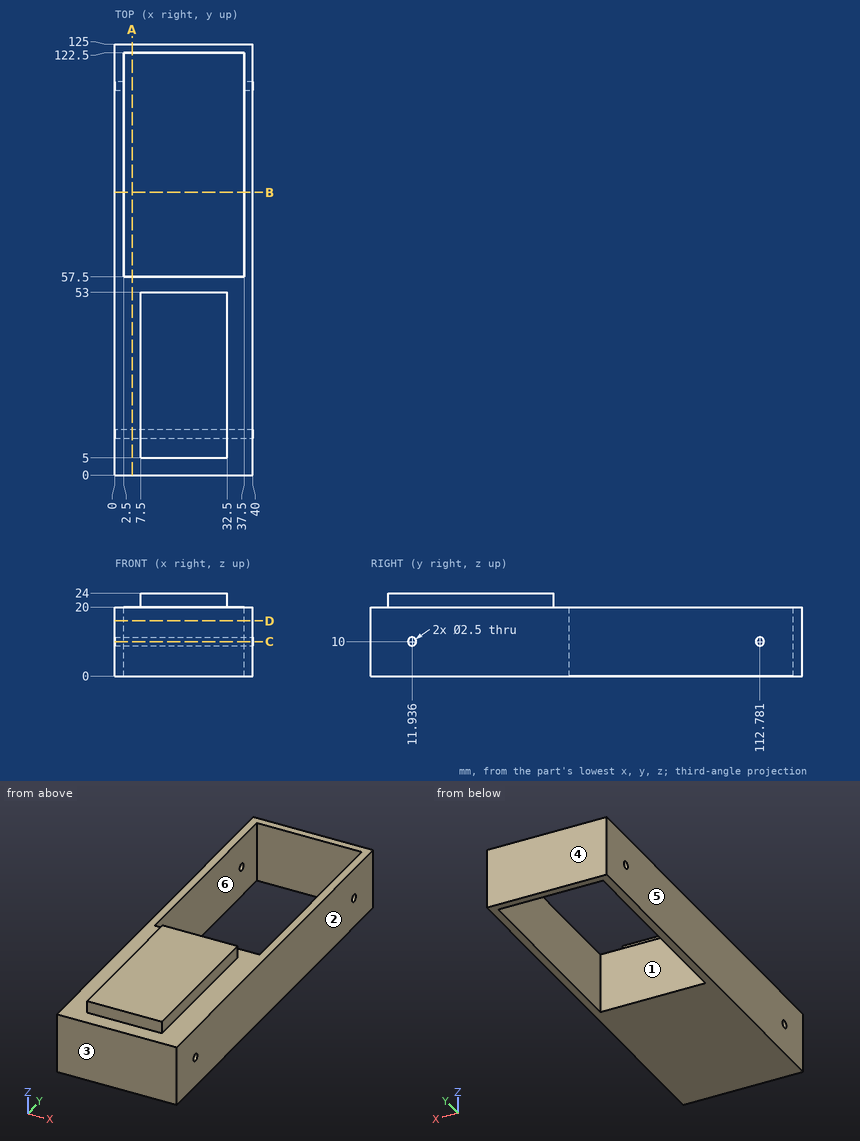
Could you check a few things on this drawing? It's one solid part, dimensions in mm from its lowest x, y, z. A direction names the side the tool comes from. Give positions to 0.01 mm unless a question says otherwise; leave off trailing zeros. Order: outer loops, then holes, each group sorted by start corner. A loop starts at its lowest first (then second) coordinate and runs counter-clockwise, first axis right, second up.
1. Thinking about a two-plate mould opening in Y: for the marked faces 3, 4, 5 and 6, which applies, +Y half, -Y half, draft (parallel to the pull), parting line (faces both ways), or undercut?
Answers below:
face 3: -Y half
face 4: +Y half
face 5: draft
face 6: undercut
2. Suppose I cut it at B-B (y = 82). Write out the boundary of the cut face in (x, z).
Answers below:
outline: (0, 0) - (2.5, 0) - (2.5, 20) - (0, 20) - close; (37.5, 0) - (40, 0) - (40, 20) - (37.5, 20) - close
3. Suppose I cut it at A-A (x = 5). Write out the boundary of the cut face in (y, z).
Answers below:
outline: (0, 0) - (57.5, 0) - (57.5, 20) - (0, 20) - close; (122.5, 0) - (125, 0) - (125, 20) - (122.5, 20) - close; hole circle Ø2.5 at (11.94, 10)
4. Suppose I cut it at C-C (z = 10). Write out the boundary of the cut face in (x, y), plus the area to 3 significant figures.
Answers below:
outline: (0, 0) - (40, 0) - (40, 10.69) - (0, 10.69) - close; (0, 13.19) - (40, 13.19) - (40, 111.53) - (37.5, 111.53) - (37.5, 57.5) - (2.5, 57.5) - (2.5, 111.53) - (0, 111.53) - close; (0, 114.03) - (2.5, 114.03) - (2.5, 122.5) - (37.5, 122.5) - (37.5, 114.03) - (40, 114.03) - (40, 125) - (0, 125) - close
area: 2,610 mm2
5. Suppose I cut it at D-D (z = 16). Write out the boundary of the cut face in (x, y).
Answers below:
outline: (0, 0) - (40, 0) - (40, 125) - (0, 125) - close; hole (2.5, 57.5) - (37.5, 57.5) - (37.5, 122.5) - (2.5, 122.5) - close
6. Which directions (+Z, -Z, +X, -X, +Y, -Y) give clear straight access to the entire face, cutting with the end or side of a thin tool? Please do the marked faces 1 and 2.
Answers below:
face 1: +Z, -Z
face 2: +Z, -Z, +X, +Y, -Y
7. For pin 1 (3 mm diameter, centred on y = 24, z = 22.5, fed in from +X); pin 2 (3 mm diameter, centred on x = 25, z = 23, fed in from -Y); pin 3 (10 mm diameter, centred on x = 6.5, y = 93, fed in from +Z), each with a flat end and sliding along its axis, tell me the tip position at first contact or that it passes through.
Answers below:
pin 1: stops at x = 32.5
pin 2: stops at y = 5
pin 3: stops at z = 20
8. I need wall thicknesses on L1, parallel to Y at x = 16.5, z = 9.75; L2, parallel to X at y = 75, z = 8; L3, parallel to Y at x = 34, z = 4.75. Which ranges of each line are inside material? Lowest first, please.
Answers below:
L1: y = 0 to 10.71, 13.16 to 57.5, 122.5 to 125
L2: x = 0 to 2.5, 37.5 to 40
L3: y = 0 to 57.5, 122.5 to 125
